Can you work these out from the model? Positions are in its coordinate system, mm. A direction names the side the tool comes from. Give positions to 0.01 mm unless a question says otherwise; leave off trailing zeros. Order: outer loops, then holes, each group sorted by start corner. A loop starts at its lowest first (then second) coordinate and runs counter-clockwise, first axis right, second up.
Item 1: I want a section at A-A, the plane z = -21.5. Write out the boundary of the cut face in (x, y).
Item 2: I want a section at C-C, the plane z = -57.5. Write out the boundary of the cut face in (x, y), then the cut area to 3 significant figures.
Item 3: If we mould it in two halves opening along Y, with no side actions, what happens to faces 5 (the flat face through (20, 184, -15.9)), 6 (the flat face through (19, -3, -19)), 7 (the flat face through (14, 184, -8)), 8 (the flat face through (19, 0, 3))? For each: +Y half, -Y half, draft (parallel to the pull), parting line (faces both ways), or undercut.
Item 4: I want a section at B-B, the plane x = -2.5. Write out the boundary of the cut face in (y, z), then the cut area to 3 significant figures.
Item 5: Which directions (+Z, -Z, +X, -X, +Y, -Y) give clear straight access to the entire face, cutting with the end or side of a thin tool? Please do faces 1 (the cylindrical face through (38, 101, -39)), 2 (the flat face through (0, 99, -20)), 3 (the flat face through (5, 195, -5)), 4 (the cylindrical face through (1, 101, -2)).
Item 6: I'm going to push flat-ended pins straight in: pin 1 Ø1.5 at (x, z) = (34.5, -6) entering from +Y; pin 2 Ø5 at (y, z) = (181, -4.5) entering from +X; pin 3 Ø2.5 at (x, z) = (-50, 25) entering from -Y; pin 4 Ø2 at (x, y) = (20, 197.5) entering from +Z. Where does each tip first touch, or does it pass through?
Item 7: If I drill on line 1 along X through (y, z) = (-1, -65); line 2 along Z through (x, y) = (-50, -1.1); line 3 along Y through (x, z) = (84, -28.5), over which ranges is the centre line in solid material (lowest first)?
```python
from build123d import *

# Parameters (mm, degrees)
SKETCH1_W               = 40
SKETCH1_H               = 40
BOSS_EXTRUDE1_DEPTH     = 200
SKETCH2_W               = 12
SKETCH2_H               = 23
CUT_EXTRUDE1_DEPTH      = 15.9
SKETCH3_R               = 1
CUT_EXTRUDE2_DEPTH      = 4
SKETCH4_R               = 5
CUT_EXTRUDE3_DEPTH      = 201
SKETCH5_W               = 13
SKETCH5_H               = 5
CUT_EXTRUDE4_DEPTH      = 4.7
SKETCH6_W               = 4
SKETCH6_H               = 10.817424305
CUT_EXTRUDE5_DEPTH      = 3
FILLET1_R               = 5
SKETCH7_W               = 150
SKETCH7_H               = 100
BOSS_EXTRUDE2_DEPTH     = 3
SKETCH9_R               = 5
CUT_EXTRUDE6_DEPTH      = 3
SKETCH10_R              = 2
CUT_EXTRUDE7_DEPTH      = 4
MIRROR2_COPY_1_SKETCH_R = 2
MIRROR2_COPY_1_DEPTH    = 4
SKETCH11_R              = 2.5
CUT_EXTRUDE8_DEPTH      = 5
MIRROR4_COPY_1_SKETCH_R = 2.5
MIRROR4_COPY_1_DEPTH    = 5
FILLET2_R               = 5


with BuildPart() as part:
    # Sketch1 → Boss-Extrude1 (new body)
    with BuildSketch(Plane(origin=(0, 0, 0), x_dir=(1, 0, 0), z_dir=(0, 1, 0))):
        with Locations((20, 20)):
            Rectangle(SKETCH1_W, SKETCH1_H)
    extrude(amount=BOSS_EXTRUDE1_DEPTH)

    # Sketch2 → Cut-Extrude1 (cut)
    with BuildSketch(Plane.XY):
        with Locations((20, 183.8)):
            Rectangle(SKETCH2_W, SKETCH2_H)
    extrude(amount=-CUT_EXTRUDE1_DEPTH, mode=Mode.SUBTRACT)

    # Sketch3 → Cut-Extrude2 (cut)
    with BuildSketch(Plane.XY):
        with Locations((20, 197.7)):
            Circle(SKETCH3_R)
        with Locations((20, 169.9)):
            Circle(SKETCH3_R)
    extrude(amount=-CUT_EXTRUDE2_DEPTH, mode=Mode.SUBTRACT)

    # Sketch4 → Cut-Extrude3 (cut, through all)
    with BuildSketch(Plane(origin=(0, 200, 0), x_dir=(1, 0, 0), z_dir=(0, 1, 0))):
        with Locations((20, 30)):
            Circle(SKETCH4_R)
    extrude(amount=-CUT_EXTRUDE3_DEPTH, mode=Mode.SUBTRACT)

    # Sketch5 → Cut-Extrude4 (cut)
    with BuildSketch(Plane(origin=(0, 200, 0), x_dir=(1, 0, 0), z_dir=(0, 1, 0))):
        with Locations((20, 12.1)):
            Rectangle(SKETCH5_W, SKETCH5_H)
    extrude(amount=-CUT_EXTRUDE4_DEPTH, mode=Mode.SUBTRACT)

    # Sketch6 → Cut-Extrude5 (cut)
    with BuildSketch(Plane(origin=(0, 200, 0), x_dir=(1, 0, 0), z_dir=(0, 1, 0))):
        with Locations((20, 20.008712153)):
            Rectangle(SKETCH6_W, SKETCH6_H)
    extrude(amount=-CUT_EXTRUDE5_DEPTH, mode=Mode.SUBTRACT)

    # Fillet1
    fillet1_edges = [part.edges().sort_by_distance(p)[0] for p in [
        (0, 100, -40),
        (40, 100, -40),
        (40, 100, 0),
        (0, 100, 0),
    ]]
    fillet(fillet1_edges, radius=FILLET1_R)

    # Sketch7 → Boss-Extrude2 (add)
    with BuildSketch(Plane.XZ):
        with Locations((20, -20)):
            Rectangle(SKETCH7_W, SKETCH7_H)
    extrude(amount=BOSS_EXTRUDE2_DEPTH)

    # Sketch9 → Cut-Extrude6 (cut)
    with BuildSketch(Plane.XZ.offset(3)):
        with Locations((20, -30)):
            Circle(SKETCH9_R)
    extrude(amount=-CUT_EXTRUDE6_DEPTH, mode=Mode.SUBTRACT)

    # Sketch10 → Cut-Extrude7 (cut, through all)
    with BuildSketch(Plane(origin=(0, 0, 0), x_dir=(1, 0, 0), z_dir=(0, 1, 0))):
        with Locations((-50, 65)):
            Circle(SKETCH10_R)
    cut_extrude7 = extrude(amount=-CUT_EXTRUDE7_DEPTH, mode=Mode.SUBTRACT)

    # Mirror1: Cut-Extrude7 across plane
    add(cut_extrude7.mirror(Plane.ZY.offset(-20)), mode=Mode.SUBTRACT)

    # Mirror2: Cut-Extrude7 across plane
    add(cut_extrude7.mirror(Plane(origin=(0, 0, -20), x_dir=(1, 0, 0), z_dir=(0, 0, -1))), mode=Mode.SUBTRACT)

    # Mirror2 copy 1 sketch → Mirror2 copy 1 (cut, through all)
    with BuildSketch(Plane(origin=(40, 0, -40), x_dir=(-1, 0, 0), z_dir=(0, 1, 0))):
        with Locations((-50, 65)):
            Circle(MIRROR2_COPY_1_SKETCH_R)
    extrude(amount=-MIRROR2_COPY_1_DEPTH, mode=Mode.SUBTRACT)

    # Sketch11 → Cut-Extrude8 (cut)
    with BuildSketch(Plane(origin=(0, 200, 0), x_dir=(1, 0, 0), z_dir=(0, 1, 0))):
        with Locations((5, 35)):
            Circle(SKETCH11_R)
    cut_extrude8 = extrude(amount=-CUT_EXTRUDE8_DEPTH, mode=Mode.SUBTRACT)

    # Mirror3: Cut-Extrude8 across plane
    add(cut_extrude8.mirror(Plane(origin=(0, 0, -20), x_dir=(1, 0, 0), z_dir=(0, 0, -1))), mode=Mode.SUBTRACT)

    # Mirror4: Cut-Extrude8 across plane
    add(cut_extrude8.mirror(Plane.ZY.offset(-20)), mode=Mode.SUBTRACT)

    # Mirror4 copy 1 sketch → Mirror4 copy 1 (cut)
    with BuildSketch(Plane(origin=(40, 200, -40), x_dir=(-1, 0, 0), z_dir=(0, 1, 0))):
        with Locations((5, 35)):
            Circle(MIRROR4_COPY_1_SKETCH_R)
    extrude(amount=-MIRROR4_COPY_1_DEPTH, mode=Mode.SUBTRACT)

    # Fillet2
    fillet2_edges = [part.edges().sort_by_distance(p)[0] for p in [
        (-55, -1.5, 30),
        (-55, -1.5, -70),
        (95, -1.5, -70),
        (95, -1.5, 30),
    ]]
    fillet(fillet2_edges, radius=FILLET2_R)


solid = part.part
```
Results list:
1. outline: (-55, -3) - (95, -3) - (95, 0) - (40, 0) - (40, 200) - (22, 200) - (22, 197) - (18, 197) - (18, 200) - (0, 200) - (0, 0) - (-55, 0) - close
2. outline: (-55, -3) - (95, -3) - (95, 0) - (-55, 0) - close
2. area: 450 mm2
3. face 5: undercut
3. face 6: -Y half
3. face 7: undercut
3. face 8: +Y half
4. outline: (-3, -70) - (0, -70) - (0, 30) - (-3, 30) - close
4. area: 300 mm2
5. face 1: -Z, +X, +Y
5. face 2: +Z, -Z, -X, +Y
5. face 3: +Y
5. face 4: +Z, -X, +Y
6. pin 1: stops at y = 195
6. pin 2: stops at x = 40
6. pin 3: passes through
6. pin 4: stops at z = 0
7. line 1: x = -55 to -52, -48 to 88, 92 to 95
7. line 2: z = -70 to -67, -63 to 23, 27 to 30
7. line 3: y = -3 to 0
